Geometry check sheet. Reference: the model listing, model coordinates, mm. Face numbers are marked on the shaded views. A direction names the side the tool comes from. Give positions to 0.01 mm unless a question says otherwise; leave off trailing zeros. Order: outer loops, then holes, each group sorted by start corner. A loop starts at its lowest first (then second) coordinate and runs counter-clockwise, first axis right, second up.
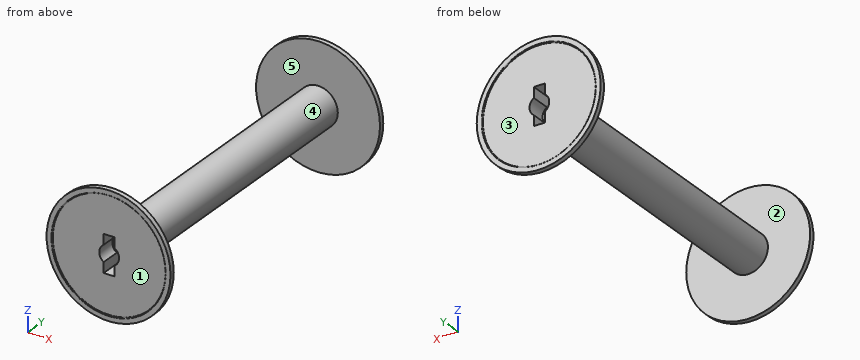
from build123d import *

# Parameters (mm, degrees)
F0_R      = 12.55
F1_DEPTH  = 1
F2_R      = 4
F3_DEPTH  = 63
F4_R      = 12.55
F5_DEPTH  = 1
F6_R      = 11.5
F7_DEPTH  = 0.2
F8_R      = 0.09999
F9_R      = 2
F10_DEPTH = 4
F11_W     = 2.25
F11_H     = 7.5
F12_DEPTH = 5
F13_R     = 11.5
F14_DEPTH = 0.2
F15_R     = 0.09999
F16_R     = 2
F17_DEPTH = 4
F18_W     = 2.25
F18_H     = 7.5
F19_DEPTH = 5


# Not quite as in the source:
# - a fillet or chamfer is up to 0.001 mm smaller than in the source, because OpenCascade refuses the exact size


with BuildPart() as f1:
    # F0 (on Front) → F1 (new body)
    with BuildSketch(Plane.XZ):
        Circle(F0_R)
    extrude(amount=F1_DEPTH)

    # F2 (on face) → F3 (join)
    with BuildSketch(Plane.XZ.offset(1)):
        Circle(F2_R)
    extrude(amount=F3_DEPTH)

    # F4 (on face) → F5 (join)
    with BuildSketch(Plane.XZ.offset(64)):
        Circle(F4_R)
    extrude(amount=F5_DEPTH)

    # F6 (on face) → F7 (cut)
    with BuildSketch(Plane.XZ.offset(65)):
        Circle(F6_R)
    extrude(amount=-F7_DEPTH, mode=Mode.SUBTRACT)

    # F8 (radius 0.1 in the source; OpenCascade refuses exactly that, so slightly less here)
    f8_edges = [f1.edges().sort_by_distance(p)[0] for p in [
        (-11.5, -65, 0),
        (11.5, -64.9, 0),
        (-11.5, -64.8, 0),
    ]]
    fillet(f8_edges, radius=F8_R)

    # F9 (on face) → F10 (cut)
    with BuildSketch(Plane.XZ.offset(64.8)):
        Circle(F9_R)
    extrude(amount=-F10_DEPTH, mode=Mode.SUBTRACT)

    # F11 (on face) → F12 (cut)
    with BuildSketch(Plane(origin=(0, -0.2, 0), x_dir=(-1, 0, 0), z_dir=(0, 1, 0))):
        Rectangle(F11_W, F11_H)
    extrude(amount=-F12_DEPTH, mode=Mode.SUBTRACT)

    # F13 (on face) → F14 (cut)
    with BuildSketch(Plane(origin=(0, 0, 0), x_dir=(-1, 0, 0), z_dir=(0, 1, 0))):
        Circle(F13_R)
    extrude(amount=-F14_DEPTH, mode=Mode.SUBTRACT)

    # F15 (radius 0.1 in the source; OpenCascade refuses exactly that, so slightly less here)
    f15_edges = [f1.edges().sort_by_distance(p)[0] for p in [
        (11.5, 0, 0),
        (11.5, -0.2, 0),
    ]]
    fillet(f15_edges, radius=F15_R)

    # F16 (on face) → F17 (cut)
    with BuildSketch(Plane(origin=(0, -0.2, 0), x_dir=(-1, 0, 0), z_dir=(0, 1, 0))):
        Circle(F16_R)
    extrude(amount=-F17_DEPTH, mode=Mode.SUBTRACT)

    # F18 (on face) → F19 (cut)
    with BuildSketch(Plane.XZ.offset(64.8)):
        Rectangle(F18_W, F18_H)
    extrude(amount=-F19_DEPTH, mode=Mode.SUBTRACT)


solid = f1.part
Item 1: Set-up check for the marked faces 1 and 2: record each of +Z, -Z, +X, -X, +Y, -Y from which the full face is reachable in a straight line by a thin tool's end or side.
Reported:
face 1: -Y
face 2: none
Item 2: Sectioned sample at A-A (y = -46). Enter the section's corners in (x, z).
Reported:
outline: circle Ø8 at (0, 0)
Item 3: Gauge pin test, flat ends, axial feed: pin 1 (5.5 mm diameter, centred on y = -1.5, z = 0, fed in from -X); pin 2 (1.1 mm diameter, centred on x = 0.5, z = 2, fed in from +Y); pin 3 (12 mm diameter, centred on y = -30.5, z = -8.5, fed in from +X); pin 4 (5 mm diameter, centred on x = 5.5, z = 0, fed in from -Y). Record the tip position at first contact, or that the pin passes through.
Reported:
pin 1: stops at x = -12.55
pin 2: stops at y = -5.2
pin 3: stops at x = 3.12
pin 4: stops at y = -64.8
Item 4: Draft check along X on the marked faces 3, 4 and 5. Enter one of: released by +X, released by -X, zero draft, split by the parting line, or undercut.
Reported:
face 3: undercut
face 4: split by the parting line
face 5: zero draft
Item 5: Scan lines: L1, parallel to Y at x = 7, z = -6.25; L2, parallel to Y at x = -7.25, z = 9; L3, parallel to Z at x = 0, y = -64.85. Record each from-to range of solid material in increasing order.
Reported:
L1: y = -64.8 to -64, -1 to -0.2
L2: y = -64.99 to -64, -1 to -0.01
L3: z = -12.55 to -11.49, 11.49 to 12.55
